Verification items for the finished model (mm, model axes). Face numbers are marked on the shaded views. A direction names the side the tool comes from. Round coordinates to 2 decimals unless told otherwise and drop trailing zeros. Loops run counter-clockwise (first coordinate to the right, second up) from the corner with the lowest first, then second, coordinate; pieces in that order, holes last. Notation, with made-up numbers: M 38.25,5.5 L 89.25,5.5 A15 cw 89.25,28.5 Z; hole C 76,-33 d3. An arc over 180 degrees is marked long. One line per item, written item: value.
from build123d import *

# Parameters (mm, degrees)
BOSS_EXTRUDE1_DEPTH = 25
SKETCH2_W           = 20
SKETCH2_H           = 3
BOSS_EXTRUDE2_DEPTH = 15
FILLET1_R           = 10
SKETCH3_R           = 1.5748
BOSS_EXTRUDE3_DEPTH = 3
SKETCH4_W           = 5
SKETCH4_H           = 5
BOSS_EXTRUDE4_DEPTH = 3.3


with BuildPart() as part:
    # Sketch1 → Boss-Extrude1 (new body)
    with BuildSketch(Plane.XY):
        Polygon((10, -3.35), (-10, -3.35), (-10, -1.35), (-1.9812, -1.35), (-1.9812, 1.35), (-10, 1.35), (-10, 3.35), (10, 3.35), (10, 1.35), (1.9812, 1.35), (1.9812, -1.35), (10, -1.35), align=None)
    extrude(amount=BOSS_EXTRUDE1_DEPTH)

    # Sketch2 → Boss-Extrude2 (add)
    with BuildSketch(Plane.XZ.offset(3.35)):
        with Locations((0, 1.5)):
            Rectangle(SKETCH2_W, SKETCH2_H)
    extrude(amount=BOSS_EXTRUDE2_DEPTH)

    # Fillet1
    fillet1_edges = [part.edges().sort_by_distance(p)[0] for p in [
        (0, -3.35, 3),
    ]]
    fillet(fillet1_edges, radius=FILLET1_R)

    # Sketch3 → Boss-Extrude3 (add)
    with BuildSketch(Plane(origin=(0, 0, 0), x_dir=(-1, 0, 0), z_dir=(0, 0, -1))):
        Circle(SKETCH3_R)
    extrude(amount=BOSS_EXTRUDE3_DEPTH)

    # Sketch4 → Boss-Extrude4 (add)
    with BuildSketch(Plane(origin=(0, 3.35, 0), x_dir=(1, 0, 0), z_dir=(0, 1, 0))):
        with Locations((0, -2.5)):
            Rectangle(SKETCH4_W, SKETCH4_H)
    extrude(amount=BOSS_EXTRUDE4_DEPTH)


solid = part.part
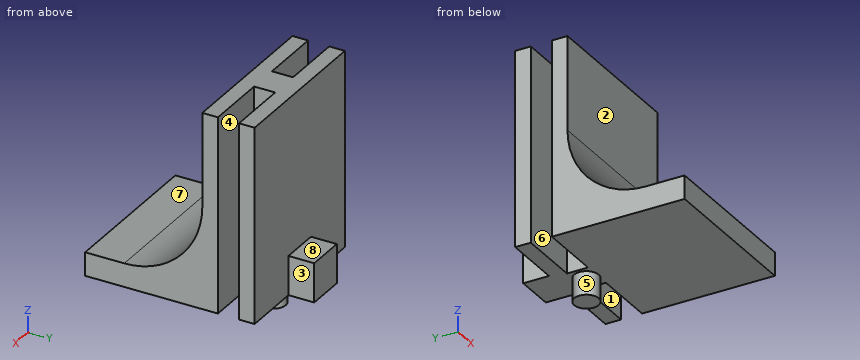
(1) Sectioned sample at B-B on z = 20.25. Enter the section's corners in (x, y), and give its area (3 significant figures).
Completed:
outline: M -10,-3.35 L 10,-3.35 L 10,-1.35 L 1.98,-1.35 L 1.98,1.35 L 10,1.35 L 10,3.35 L -10,3.35 L -10,1.35 L -1.98,1.35 L -1.98,-1.35 L -10,-1.35 Z
area: 90.7 mm^2
(2) Thickness scan on L1, parallel to Y at x = 3.25, z = 20.5; L2, parallel to Z at x = 8.25, y = -3. Record the ranges inside material, lowest first. Write a range as from..to.
Completed:
L1: y = -3.35..-1.35, 1.35..3.35
L2: z = 0..25
(3) Sectioned sample at A-A on x = -8. Enter the section's corners in (y, z).
Completed:
outline: M -18.35,0 L -1.35,0 L -1.35,25 L -3.35,25 L -3.35,13 A10 cw -13.35,3 L -18.35,3 Z; M 1.35,0 L 3.35,0 L 3.35,25 L 1.35,25 Z
(4) Sectioned sample at C-C on x = 0. Enter the section's corners in (y, z), and give its area (3 significant figures).
Completed:
outline: M -18.35,0 L -1.57,0 L -1.57,-3 L 1.57,-3 L 1.57,0 L 6.65,0 L 6.65,5 L 3.35,5 L 3.35,25 L -3.35,25 L -3.35,13 A10 cw -13.35,3 L -18.35,3 Z
area: 260 mm^2
(5) Mould release check, pull along Y, two halves, no side actions. Record for the marked faces 1, 2 and 3: +Y half, -Y half, draft (parallel to the pull), parting line (faces both ways), or undercut.
Completed:
face 1: undercut
face 2: -Y half
face 3: draft
(6) Tool access check on the marked faces 4, 5, 6, 7 and 8. Record the directions out of +Z, -Z, +X, -X, +Y, -Y that give a thin tool (end or side, any length) a straight path to the whole face; none if there is none.
Completed:
face 4: +Z, -Z, +X
face 5: -Z
face 6: +Z, -Z, -X
face 7: +Z, +X, -X, -Y
face 8: +Z, +X, -X, +Y
(7) Sectioned sample at D-D on y = 0. Enter the section's corners in (x, z), and give its area (3 significant figures).
Completed:
outline: M -1.98,0 L -1.57,0 L -1.57,-3 L 1.57,-3 L 1.57,0 L 1.98,0 L 1.98,25 L -1.98,25 Z
area: 109 mm^2
(8) Depth check by flat-ended pin: pin 1 Ø1.5 at (x, z) = (-4.5, 10) entering from -Y; pin 2 Ø4 at (x, z) = (6, 16.5) entering from -Y; pin 3 Ø5.5 at (x, y) = (1, -16.5) entering from +Z; pin 4 Ø3.5 at (y, z) = (4.5, 3) entering from +X. Enter the tip coordinate at first touch or a pass-through.
Completed:
pin 1: stops at y = -4.08
pin 2: stops at y = -3.35
pin 3: stops at z = 3
pin 4: stops at x = 10
